Build history of the part. All positions in model axes, mm. Coordinates: 2 decimals unless noted, no trailing zeros. Loops run counter-clockwise (first coordinate to the right, second up) from the corner with the lowest first, then second, coordinate; pieces in that order, holes last.
(1) Slice it at B-B (z = 8). Give the cut face in (x, y), and give its area (3 significant figures).
(2) Slice it at D-D (y = 149.5). Give the cut face in (x, z), and give its area (3 significant figures).
(3) Flat gauge pins, fed straight in: P1, Ø4, axis at x = 47, y = 59, coming from the +Z side; P2, Ø5, axis at x = 79, z = -91.5, coming from the -Y side; P3, Ø10, axis at x = 30, z = 123.5, coming from the +Y side; P4, Ø3, axis at y = 14, z = -42.5, coming from the -X side. Where does each tip first touch, or does it go through?
(4) Slice it at A-A (y = 111.5). Give the cut face in (x, z).
(5) Slice it at C-C (x = 38). Give the cut face in (y, z), and give its area (3 significant figures).
(6) Two-plate mould, pull along Z, no slides. Class faces 1 (the face through (53.55, 42.81, -78.07)), 2 (the face through (40, -62.859, 13)): pulls with the +Z half, pulls with the -Z half, needs draft (parallel to the pull), parting line crosses it, or undercut.
(7) Wall check: L1, parallel to Y at x = 37.5, z = 0; L2, parallel to Z at x = 82, y = 125.5; L3, parallel to Z at x = 84, y = 112. Give the ranges that are in metal, low to high.
from build123d import *

# Parameters (mm, degrees)
F0_W      = 105.6232824922
F0_H      = 62.8593713045
F1_DEPTH  = 25.4
F1_FACE_W = 105.6232824922
F1_FACE_H = 62.8593713045
F5_DEPTH  = 25.4


with BuildPart() as f1:
    # F0 (on Top) → F1 (new body)
    with BuildSketch(Plane.XY):
        with Locations((52.8116412461, -31.4296856523)):
            Rectangle(F0_W, F0_H)
    extrude(amount=F1_DEPTH)

    # F1_face (on face) → F3 (revolve)
    with BuildSketch(Plane(origin=(52.8116412461, -31.4296856523, 0), x_dir=(1, 0, 0), z_dir=(0, 0, -1))):
        Rectangle(F1_FACE_W, F1_FACE_H)
    revolve(axis=Axis((0, 92.5896167755, 0), (1, 0, 0)))

    # F4 (on face) → F5 (cut)
    with BuildSketch(Plane.YZ.offset(105.6232824922)):
        with BuildLine():
            ThreePointArc((-62.8593713045, 0), (-62.3361935892, 12.742887347), (-60.7701820477, 25.4))
            Line((-60.7701820477, 25.4), (-62.8593713045, 25.4))
            Line((-62.8593713045, 25.4), (-62.8593713045, 0))
        make_face()
    extrude(amount=-F5_DEPTH, mode=Mode.SUBTRACT)


solid = f1.part
Response values:
1. outline: (0, -62.86) - (80.22, -62.86) - (80.22, -62.65) - (105.62, -62.65) - (105.62, 0.35) - (0, 0.35) - close; (0, 184.83) - (105.62, 184.83) - (105.62, 247.83) - (0, 247.83) - close
1. area: 13,300 mm2
2. outline: (0, -144.66) - (105.62, -144.66) - (105.62, -73.03) - (0, -73.03) - close; (0, 73.03) - (105.62, 73.03) - (105.62, 144.66) - (0, 144.66) - close
2. area: 15,100 mm2
3. P1: stops at z = 152.21
3. P2: stops at y = -34.86
3. P3: stops at y = 193.2
3. P4: passes through
4. outline: (0, -154.29) - (105.62, -154.29) - (105.62, -90.64) - (0, -90.64) - close; (0, 90.64) - (105.62, 90.64) - (105.62, 154.29) - (0, 154.29) - close
5. outline: (-62.86, 0) arc R155.45 ccw (long way) to (-60.77, 25.4) - (-62.86, 25.4) - close; hole circle Ø185.18 at (92.59, 0)
5. area: 49,000 mm2
6. face 1: undercut
6. face 2: needs draft
7. L1: y = -62.86 to 0, 185.18 to 248.04
7. L2: z = -151.93 to -86.54, 86.54 to 151.93
7. L3: z = -154.23 to -90.53, 90.53 to 154.23
